Here's how the part is built. I have some questions about the finished solid (model axes, mm). Face numbers are marked on the shaded views. Round coordinates to 2 decimals unless told otherwise and drop trailing zeros. Write each loop counter-clockwise with the first axis right and the second up, starting at its lowest first coordinate (ties: lowest second). Pieces come first, ordered by that corner, then holes. Notation, with made-up numbers: (49, 63) -> (72, 63) arc R27 cw to (72, 96) -> close; hole circle Ø10 at (10.5, 64.25). An arc over 180 degrees is marked (long way). Put each result on its own line as item: value. Start each with the question number.
1. Suppose I cut it at C-C (y = -26.5). Please give me the cut outline in (x, z).
2. Suppose I cut it at A-A (y = -1.5). Please give me the cut outline in (x, z).
3. Suppose I cut it at B-B (z = 9). Count the separate pieces of the cut face and the enclosed holes in it, then the cut area to 3 significant figures.
4. We'd pull the mould along Z, two halves only. Please class the marked faces 1, 2 and 3: +Z half, -Z half, draft (parallel to the pull), parting line (faces both ways), or undercut.
5. For pin 1 (10 mm diameter, centred on x = -9, y = -24, fed in from +Z); pin 2 (8 mm diameter, centred on x = -1.5, z = 7, fed in from -Y); pin 3 (1 mm diameter, centred on y = -23, z = -12.5, fed in from -X), each with a flat end and sliding along its axis, tell me the tip position at first contact or that it passes through.
6. I need wall thicknesses on probe 1 along Y at (x, z) = (-31.5, 9); probe 2 along Z at (x, y) = (-60, 4.5); probe 3 along Z at (x, y) = (7.5, 9). Which ranges of each line are inside material? Lowest first, please. Write a range as from..to.
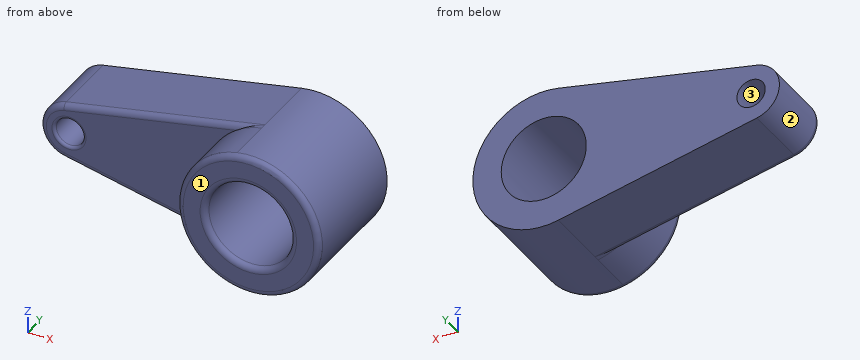
```python
from build123d import *

# Parameters (mm, degrees)
F0_R         = 15
F0_R_2       = 5
F1_DEPTH     = 12.5
F2_DEPTH     = 30
F3_T4_DEPTH  = 86.5228675813
F3_S5_R      = 25
F3_T6_DEPTH  = 45
F3_T8_ANGLE  = 156.3108298238
F3_T12_DEPTH = 86.5228675813
F3_S13_R     = 25
F3_T14_DEPTH = 45
F4_R         = 1


# Not quite as in the source:
# - a fillet or chamfer that OpenCascade refuses, or shapes differently, is made with other operations: its cross-section is extruded or revolved along the edge and cut away or added


with BuildPart() as f1:
    # F0 (on Front) → F1 (new body, symmetric)
    with BuildSketch(Plane.XZ):
        with BuildLine():
            ThreePointArc((-60.0797491716, 17.2713649638), (-51.7234339832, 15.247202645), (-48.0271721521, 7.4842853392))
            ThreePointArc((-48.0271721521, 7.4842853392), (-51.7234339832, -0.2786319667), (-60.0797491716, -2.3027942855))
            Line((-60.0797491716, -2.3027942855), (9.9202508284, -16.9834137224))
            ThreePointArc((9.9202508284, -16.9834137224), (-9.9483066228, 7.4842853392), (9.9202508284, 31.9519844007))
            Line((9.9202508284, 31.9519844007), (-60.0797491716, 17.2713649638))
        make_face()
        with BuildLine():
            ThreePointArc((40.0516933772, 7.4842853392), (30.8110387995, 26.8915786038), (9.9202508284, 31.9519844007))
            ThreePointArc((9.9202508284, 31.9519844007), (-9.9483066228, 7.4842853392), (9.9202508284, -16.9834137224))
            ThreePointArc((9.9202508284, -16.9834137224), (30.8110387995, -11.9230079255), (40.0516933772, 7.4842853392))
        make_face()
        with Locations((15.0516933772, 7.4842853392)):
            Circle(F0_R, mode=Mode.SUBTRACT)
        with BuildLine():
            ThreePointArc((-60.0797491716, -2.3027942855), (-51.7234339832, -0.2786319667), (-48.0271721521, 7.4842853392))
            ThreePointArc((-48.0271721521, 7.4842853392), (-51.7234339832, 15.247202645), (-60.0797491716, 17.2713649638))
            ThreePointArc((-60.0797491716, 17.2713649638), (-68.0271721521, 7.4842853392), (-60.0797491716, -2.3027942855))
        make_face()
        with Locations((-58.0271721521, 7.4842853392)):
            Circle(F0_R_2, mode=Mode.SUBTRACT)
    extrude(amount=F1_DEPTH, both=True)

    # F0 (on Front) → F2 (join)
    with BuildSketch(Plane.XZ):
        with BuildLine():
            ThreePointArc((40.0516933772, 7.4842853392), (30.8110387995, 26.8915786038), (9.9202508284, 31.9519844007))
            ThreePointArc((9.9202508284, 31.9519844007), (-9.9483066228, 7.4842853392), (9.9202508284, -16.9834137224))
            ThreePointArc((9.9202508284, -16.9834137224), (30.8110387995, -11.9230079255), (40.0516933772, 7.4842853392))
        make_face()
        with Locations((15.0516933772, 7.4842853392)):
            Circle(F0_R, mode=Mode.SUBTRACT)
    extrude(amount=F2_DEPTH)

    # F3: fillet of radius 2 on 5 edges, made by hand


with BuildPart() as f3_tool2:
    # F3_s3 → F3_t4 (new body)
    with BuildSketch(Plane(origin=(-57.0859435933, 0, 11.9722430442), x_dir=(0, 1, 0), z_dir=(0.9787079625, 0, -0.205257702))):
        with BuildLine():
            ThreePointArc((-12.5, -12.5855943521), (-11.9142135624, -13.9998079144), (-10.5, -14.5855943521))
            Line((-10.5, -14.5855943521), (-12.5, -14.5855943521))
            Line((-12.5, -14.5855943521), (-12.5, -12.5855943521))
        make_face()
    extrude(amount=F3_T4_DEPTH)

    # F3_s5 → F3_t6 (cut, symmetric)
    with BuildSketch(Plane.XZ.offset(11.5)):
        with Locations((15.0516933772, 7.4842853392)):
            Circle(F3_S5_R)
    extrude(amount=F3_T6_DEPTH, both=True, mode=Mode.SUBTRACT)


with BuildPart() as f1_1:
    add(f1.part)

    # F3_t1: cut F3_tool2
    add(f3_tool2.part, mode=Mode.SUBTRACT)

    # F3_s7 → F3_t8 (revolve, cut)
    with BuildSketch(Plane(origin=(-54.0789471374, 0, -11.3416063211), x_dir=(0, 1, 0), z_dir=(0.9787079625, 0, 0.205257702))):
        with BuildLine():
            ThreePointArc((-10.5, 29.2354536617), (-11.9142135624, 28.649667224), (-12.5, 27.2354536617))
            Line((-12.5, 27.2354536617), (-12.5, 29.2354536617))
            Line((-12.5, 29.2354536617), (-10.5, 29.2354536617))
        make_face()
    revolve(axis=Axis((-58.0271721521, -12.5, 7.4842853392), (0, -1, 0)), revolution_arc=F3_T8_ANGLE, mode=Mode.SUBTRACT)


with BuildPart() as f3_tool10:
    # F3_s11 → F3_t12 (new body)
    with BuildSketch(Plane(origin=(30.6016722995, 0, 6.4178786452), x_dir=(0, 1, 0), z_dir=(-0.9787079625, 0, -0.205257702))):
        with BuildLine():
            ThreePointArc((-10.5, -29.2354536617), (-11.9142135624, -28.649667224), (-12.5, -27.2354536617))
            Line((-12.5, -27.2354536617), (-12.5, -29.2354536617))
            Line((-12.5, -29.2354536617), (-10.5, -29.2354536617))
        make_face()
    extrude(amount=F3_T12_DEPTH)

    # F3_s13 → F3_t14 (cut, symmetric)
    with BuildSketch(Plane.XZ.offset(11.5)):
        with Locations((15.0516933772, 7.4842853392)):
            Circle(F3_S13_R)
    extrude(amount=F3_T14_DEPTH, both=True, mode=Mode.SUBTRACT)


with BuildPart() as f1_2:
    add(f1_1.part)

    # F3_t9: cut F3_tool10
    add(f3_tool10.part, mode=Mode.SUBTRACT)

    # F3_s15 → F3_t16 (revolve, cut)
    with BuildSketch(Plane(origin=(15.9210528626, 0, 3.3390131159), x_dir=(0, 1, 0), z_dir=(-0.9787079625, 0, -0.205257702))):
        with BuildLine():
            ThreePointArc((-28, -29.2354536617), (-29.4142135624, -28.649667224), (-30, -27.2354536617))
            Line((-30, -27.2354536617), (-30, -29.2354536617))
            Line((-30, -29.2354536617), (-28, -29.2354536617))
        make_face()
    revolve(axis=Axis((15.0516933772, -30, 7.4842853392), (0, 1, 0)), mode=Mode.SUBTRACT)

    # F3_s17 → F3_t18 (revolve, cut)
    with BuildSketch(Plane.XY.offset(7.4842853392)):
        with BuildLine():
            ThreePointArc((32.0516933772, -30), (30.6374798149, -29.4142135624), (30.0516933772, -28))
            Line((30.0516933772, -28), (30.0516933772, -30))
            Line((30.0516933772, -30), (32.0516933772, -30))
        make_face()
    revolve(axis=Axis((15.0516933772, -30, 7.4842853392), (0, -1, 0)), mode=Mode.SUBTRACT)

    # F4
    f4_edges = [f1_2.edges().sort_by_distance(p)[0] for p in [
        (-63.027172, -12.5, 7.484285),
    ]]
    fillet(f4_edges, radius=F4_R)


solid = f1_2.part
```
Verdict:
1. outline: circle Ø50 at (15.05, 7.48); hole circle Ø30 at (15.05, 7.48)
2. outline: (-60.08, -2.3) -> (9.92, -16.98) arc R25 ccw (long way) to (9.92, 31.95) -> (-60.08, 17.27) arc R10 ccw to start; hole circle Ø10 at (-58.03, 7.48); hole circle Ø30 at (15.05, 7.48)
3. separate pieces: 3
3. enclosed holes: 0
3. area: 2,060 mm^2
4. face 1: draft
4. face 2: parting line
4. face 3: undercut
5. pin 1: stops at z = 23.67
5. pin 2: stops at y = -30
5. pin 3: stops at x = -0.61
6. probe 1: y = -12.5..12.5
6. probe 2: z = -2.32..2.89, 12.08..17.29
6. probe 3: z = -16.48..-5.48, 20.44..31.44
